```python
from build123d import *

# Parameters (mm, degrees)
BOSS_EXTRUDE1_DEPTH = 31
SKETCH2_R           = 1.5025
CUT_EXTRUDE1_DEPTH  = 6.005
SKETCH3_R           = 1.5025
CUT_EXTRUDE2_DEPTH  = 3.005


with BuildPart() as part:
    # Sketch1 → Boss-Extrude1 (new body)
    with BuildSketch(Plane(origin=(0, 0, 0), x_dir=(1, 0, 0), z_dir=(0, 1, 0))):
        Polygon((2.5, 1.443375673), (0, 2.886751346), (-2.5, 1.443375673), (-2.5, -1.443375673), (0, -2.886751346), (2.5, -1.443375673), align=None)
    extrude(amount=BOSS_EXTRUDE1_DEPTH)

    # Sketch2 → Cut-Extrude1 (cut)
    with BuildSketch(Plane(origin=(0, 0, 0), x_dir=(1, 0, 0), z_dir=(0, 1, 0))):
        Circle(SKETCH2_R)
    extrude(amount=CUT_EXTRUDE1_DEPTH, mode=Mode.SUBTRACT)

    # Sketch3 → Cut-Extrude2 (cut)
    with BuildSketch(Plane(origin=(0, 31, 0), x_dir=(1, 0, 0), z_dir=(0, 1, 0))):
        Circle(SKETCH3_R)
    extrude(amount=-CUT_EXTRUDE2_DEPTH, mode=Mode.SUBTRACT)


solid = part.part
```
Work out the finished part from the listing and answer in its coordinate system (mm). A direction names the side the tool comes from. Round coordinates to 2 decimals unless told otherwise and drop trailing zeros. Write each loop counter-clockwise with the first axis right and the second up, starting at its lowest first coordinate (ties: lowest second). Pieces come first, ordered by that corner, then holes. Notation, with made-up numbers: (1, 79.5) -> (58, 79.5) arc R8 cw to (58, 88.5) -> close; hole circle Ø9 at (78, -5). An arc over 180 degrees is marked (long way). Write each question's results on one line, items separated by ' | '.
Q1. Which of the six approach directions +Z, -Z, +X, -X, +Y, -Y give full straight-line access (tool end or side, diameter ignored) to faces 4 (the flat face through (-1.15, 31, 1.24)), 5 (the cylindrical face through (1.433, 2.96, -0.451)), 6 (the flat face through (0, 27.995, 0))?
Data:
face 4: +Z, -Z, +X, -X, +Y | face 5: -Y | face 6: +Y
Q2. Section C-C, the plane x = -1.15 is taken. Write down the section's boundary in (y, z) (3 decimals).
Data:
outline: (0, -2.223) -> (31, -2.223) -> (31, -0.967) -> (27.995, -0.967) -> (27.995, 0.967) -> (31, 0.967) -> (31, 2.223) -> (0, 2.223) -> (0, 0.967) -> (6.005, 0.967) -> (6.005, -0.967) -> (0, -0.967) -> close
Q3. Section A-A, the plane y = 2.5 is taken. Write down the section's boundary in (x, z) (1 decimal).
Data:
outline: (-2.5, -1.4) -> (0, -2.9) -> (2.5, -1.4) -> (2.5, 1.4) -> (0, 2.9) -> (-2.5, 1.4) -> close; hole circle Ø3 at (0, 0)
Q4. Flat-ended cylindrical pins translate along their axes: P1, Ø1.8, axis at x = 0, z = 0, coming from the +Y side (3 decimals); P2, Ø3, axis at x = 0, y = 16, coming from the -Z side; P3, Ø1, axis at x = 1, y = 12, coming from the +Z side. Find the tip coordinate at first contact, or state that the pin passes through.
Data:
P1: y = 27.995 | P2: z = -2.89 | P3: z = 2.6
Q5. Section D-D, the plane y = 14.5 is taken. Write down the section's boundary in (x, z), then the cut area to 3 significant figures.
Data:
outline: (-2.5, -1.44) -> (0, -2.89) -> (2.5, -1.44) -> (2.5, 1.44) -> (0, 2.89) -> (-2.5, 1.44) -> close | area: 21.7 mm^2
Q6. Section B-B, the plane z = 0 is taken. Write down the section's boundary in (x, y) (1 decimal).
Data:
outline: (-2.5, 0) -> (-1.5, 0) -> (-1.5, 6) -> (1.5, 6) -> (1.5, 0) -> (2.5, 0) -> (2.5, 31) -> (1.5, 31) -> (1.5, 28) -> (-1.5, 28) -> (-1.5, 31) -> (-2.5, 31) -> close
Q7. Determine the mould class of faces 1 (the flat face through (2.5, 15, 0)), 2 (the flat face through (0, 6.005, 0)), 3 (the flat face through (-2.5, 15, 0)) for opening direction X: released by +X, released by -X, zero draft, split by the parting line, or undercut.
Data:
face 1: released by +X | face 2: undercut | face 3: released by -X
Q8. Straight lines are drawn through the part: line 1 along X through (y, z) = (30.35, 0); line 2 along Y through (x, z) = (1.15, 0.65) (3 decimals); line 3 along X through (y, z) = (3.5, 0.8). For each, find the intervals that lie inside material, in ascending order. Write a range as [from, to].
Data:
line 1: [-2.5, -1.5], [1.5, 2.5] | line 2: [6.005, 27.995] | line 3: [-2.5, -1.27], [1.27, 2.5]
